```python
from build123d import *

# Parameters (mm, degrees)
SKETCH1_W           = 47
SKETCH1_H           = 40
SKETCH1_R           = 2.1
BOSS_EXTRUDE1_DEPTH = 40
SKETCH6_OUTSIDE_W   = 63.71
SKETCH6_OUTSIDE_H   = 56.71
SKETCH6_OUTSIDE_W_2 = 47
SKETCH6_OUTSIDE_H_2 = 40
SKETCH6_OUTSIDE_R   = 15
CUT_EXTRUDE5_DEPTH  = 71.455659815
CUT_EXTRUDE6_DEPTH  = 71.455659815


with BuildPart() as part:
    # Sketch1 → Boss-Extrude1 (new body)
    with BuildSketch(Plane.XY):
        with Locations((18.5, 15)):
            Rectangle(SKETCH1_W, SKETCH1_H)
        Circle(SKETCH1_R, mode=Mode.SUBTRACT)
        with Locations((37, 0)):
            Circle(SKETCH1_R, mode=Mode.SUBTRACT)
        with Locations((0, 30)):
            Circle(SKETCH1_R, mode=Mode.SUBTRACT)
        with Locations((37, 30)):
            Circle(SKETCH1_R, mode=Mode.SUBTRACT)
    extrude(amount=BOSS_EXTRUDE1_DEPTH)

    # Sketch6 outside → Cut-Extrude5 (cut, through all)
    # profile 1 of 2: a face of its own
    with BuildSketch(Plane(origin=(0, 35, 0), x_dir=(1, 0, 0), z_dir=(0, 1, 0))):
        with Locations((18.5, -20)):
            Rectangle(SKETCH6_OUTSIDE_W, SKETCH6_OUTSIDE_H)
        with Locations((18.5, -20)):
            Rectangle(SKETCH6_OUTSIDE_W_2, SKETCH6_OUTSIDE_H_2, mode=Mode.SUBTRACT)
    # profile 2 of 2: a face of its own
    with BuildSketch(Plane(origin=(0, 35, 0), x_dir=(1, 0, 0), z_dir=(0, 1, 0))):
        with Locations(Location((18.5, -20, 0), (0, 0, 270))):
            Circle(SKETCH6_OUTSIDE_R)
    extrude(amount=-CUT_EXTRUDE5_DEPTH, mode=Mode.SUBTRACT)

    # Sketch7 → Cut-Extrude6 (cut, through all)
    with BuildSketch(Plane(origin=(0, 35, 0), x_dir=(1, 0, 0), z_dir=(0, 1, 0))):
        with BuildLine():
            Line((33.5, -20), (42, -20))
            Line((42, -20), (42, -18))
            Line((42, -18), (33.366068747, -18))
            ThreePointArc((33.366068747, -18), (33.466479733, -18.997760311), (33.5, -20))
        make_face()
        with BuildLine():
            Line((42, -22), (42, -20))
            Line((42, -20), (33.5, -20))
            ThreePointArc((33.5, -20), (33.466479733, -21.002239689), (33.366068747, -22))
            Line((33.366068747, -22), (42, -22))
        make_face()
    extrude(amount=-CUT_EXTRUDE6_DEPTH, mode=Mode.SUBTRACT)


solid = part.part
```
Could you check a few things on this model? Use its own coordinates, in mm. A direction names the side the tool comes from. Round coordinates to 2 decimals unless told otherwise and drop trailing zeros. Loops run counter-clockwise (first coordinate to the right, second up) from the corner with the lowest first, then second, coordinate; pieces in that order, holes last. Notation, with made-up numbers: (26.25, -38.75) - (83.25, -38.75) arc R29 ccw to (83.25, 0.25) - close; hole circle Ø1 at (-12.75, -34). An arc over 180 degrees is marked (long way). Answer in a Markdown table with one row per item. Add a question column.
(1) If we section it at B-B (z = 23): Please give me the cut outline in (x, y).
(2) I need wall thicknesses on line 1 along Y through (x, z) = (0, 30); line 2 along X through (y, z) = (29.5, 25.5); line 3 along Z through (x, y) = (38, 12.5). Which ranges of each line are inside material? Lowest first, please.
(3) I'm going to push flat-ended pins straight in: pin 1 (5.5 mm diameter, centred on x = 37, y = 30, fed in from +Z); pin 2 (1 mm diameter, centred on y = 0.5, z = 21, fed in from +X). Where does each tip first touch, or does it pass through?
(4) If we section it at D-D (y = 0): Please give me the cut outline in (x, z).
(5) If we section it at C-C (x = 0): Please give me the cut outline in (y, z), plus the area to 3 significant figures.
(6) If we mould it in two halves opening along Y, with no side actions, what happens to faces 1 (the face through (3, -5, 20)), 2 (the face through (34.9, 0.09, 30.87)), 3 (the face through (18, 15, 40)), 4 (the face through (34.9, 0.09, 8.87))? For each: pulls with the +Y half, pulls with the -Y half, needs draft (parallel to the pull), parting line crosses it, or undercut.
(7) If we section it at A-A (x = 18.5): Please give me the cut outline in (y, z).
(8) For faces 5 (the face through (38, 15, 22)), 6 (the face through (42, 15, 31)), which set-ups out of +Z, -Z, +X, -X, +Y, -Y let a thin tool reach every point of the face, with its end or its side?
Model answer:
| question | item | result |
|---|---|---|
| 1 | outline | (-5, -5) - (3.8, -5) - (3.8, 35) - (-5, 35) - close; (33.2, -5) - (42, -5) - (42, 35) - (33.2, 35) - close; hole circle Ø4.2 at (0, 0); hole circle Ø4.2 at (0, 30); hole circle Ø4.2 at (37, 0); hole circle Ø4.2 at (37, 30) |
| 2 | line 1 | y = -5 to -2.1, 2.1 to 27.9, 32.1 to 35 |
| 2 | line 2 | x = -5 to -2.04, 2.04 to 4.54, 32.46 to 34.96, 39.04 to 42 |
| 2 | line 3 | z = 0 to 18, 22 to 40 |
| 3 | pin 1 | stops at z = 40 |
| 3 | pin 2 | stops at x = 3.58 |
| 4 | outline | (-5, 0) - (-2.1, 0) - (-2.1, 40) - (-5, 40) - close; (2.1, 0) - (34.9, 0) - (34.9, 18) - (33.37, 18) arc R15 cw (long way) to (33.37, 22) - (34.9, 22) - (34.9, 40) - (2.1, 40) - close; (39.1, 0) - (42, 0) - (42, 18) - (39.1, 18) - close; (39.1, 22) - (42, 22) - (42, 40) - (39.1, 40) - close |
| 5 | outline | (-5, 0) - (-2.1, 0) - (-2.1, 40) - (-5, 40) - close; (2.1, 0) - (27.9, 0) - (27.9, 40) - (2.1, 40) - close; (32.1, 0) - (35, 0) - (35, 40) - (32.1, 40) - close |
| 5 | area | 1,260 mm² |
| 6 | face 1 | pulls with the -Y half |
| 6 | face 2 | undercut |
| 6 | face 3 | needs draft |
| 6 | face 4 | undercut |
| 7 | outline | (-5, 0) - (35, 0) - (35, 5) - (-5, 5) - close; (-5, 35) - (35, 35) - (35, 40) - (-5, 40) - close |
| 8 | face 5 | +X, +Y, -Y |
| 8 | face 6 | +Z, -Z, +X, +Y, -Y |
